For this review, use the dimensioned drawing (mm, ordinates from the lowest corner) and the shaded views. A direction names the side the tool comes from. Round coordinates to 2 decimals unless told otherwise and drop trailing zeros. Loops run counter-clockwise (first coordinate to the right, second up) from the corner with the lowest first, then second, coordinate; pieces in that order, holes last. Notation, with made-up numbers: M -3.75,42.25 L 49.25,42.25 A33 cw 49.25,79.25 Z; hole C 86.5,-36.5 d10. An arc over 180 degrees is marked long. One line per item, written item: value. Start each with the question number.
Item 1: For line 1 along Y through (x, z) = (5.5, 7.25); line 2 along X through (y, z) = (25.5, 5.5); line 3 along X through (y, z) = (42.5, 3.5), list the stretches that pass through material, from the lowest coordinate up.
Item 2: We need section A-A (z = 5.5). Write out the cut boundary in (x, y).
Item 3: We need section D-D (y = 42.5). Write out the cut boundary in (x, z).
Item 4: Clearance check with flat-ended pins moving along their axes: pin 1 (6 mm diameter, centred on y = 23, z = 8, fed in from +X); pin 2 (2 mm diameter, centred on y = 36, z = 2.5, fed in from +X); pin 3 (1.8 mm diameter, centred on x = 5.5, y = 42.5, fed in from -Z); pin 4 (3 mm diameter, centred on x = 1.5, y = 13, fed in from +Z). State where each tip first meets the part, or that it passes through.
Item 5: For the marked faces 1, 2 and 3, list the 3-axis set-ups (+Z, -Z, +X, -X, +Y, -Y) from which the entire face can be reached by the end or side of a thin tool; tool diameter is ignored.
Item 6: We need section B-B (x = 5.5). Write out the cut boundary in (y, z), then the cut area to 3 significant figures.
Item 7: We need section C-C (y = 11). Write out the cut boundary in (x, z).
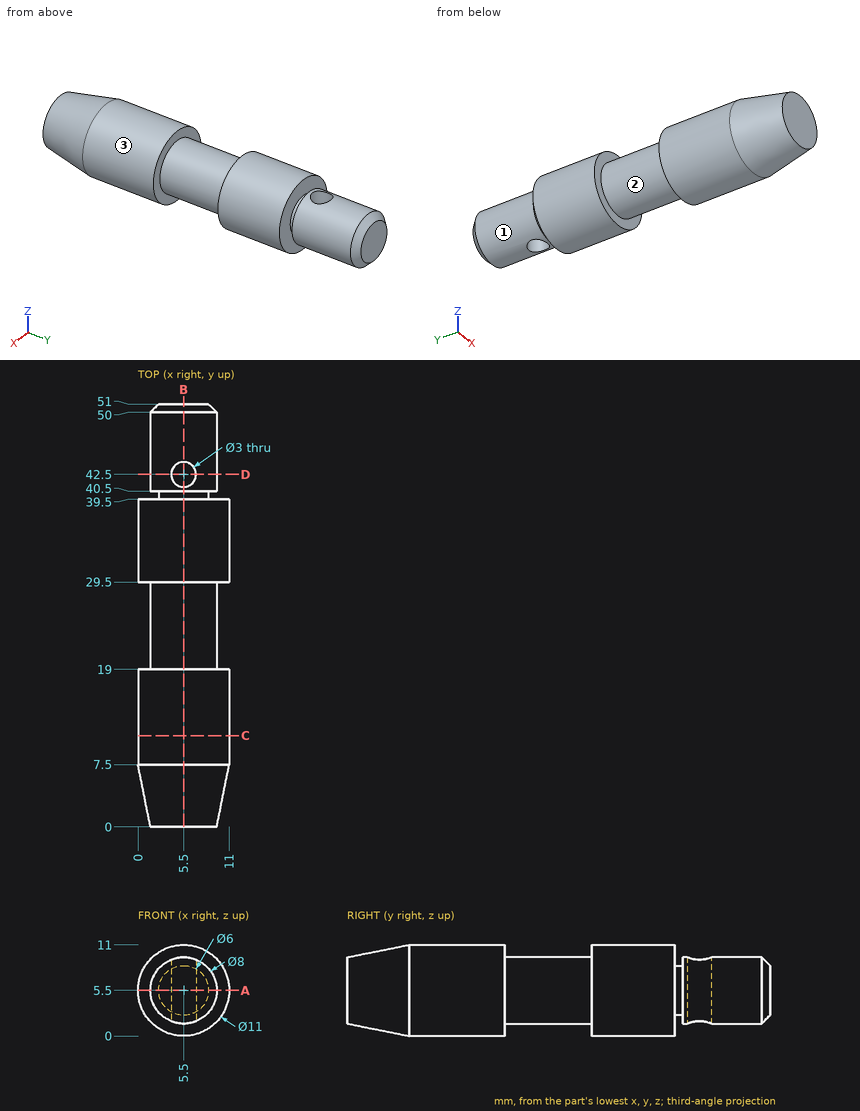
A:
1. line 1: 0 to 41, 44 to 51
1. line 2: 1.5 to 9.5
1. line 3: 2.04 to 4, 7 to 8.96
2. outline: M 0,7.5 L 1.5,0 L 9.5,0 L 11,7.5 L 11,19 L 9.5,19 L 9.5,29.5 L 11,29.5 L 11,39.5 L 8.5,39.5 L 8.5,40.5 L 9.5,40.5 L 9.5,50 L 8.5,51 L 2.5,51 L 1.5,50 L 1.5,40.5 L 2.5,40.5 L 2.5,39.5 L 0,39.5 L 0,29.5 L 1.5,29.5 L 1.5,19 L 0,19 Z; hole C 5.5,42.5 d3
3. outline: M 4,1.79 L 4,9.21 A4 ccw Z; M 7,1.79 A4 ccw 7,9.21 Z
4. pin 1: x = 9.5
4. pin 2: x = 10.62
4. pin 3: through
4. pin 4: z = 10.4
5. face 1: +Y
5. face 2: none
5. face 3: +Y, -Y
6. outline: M 0,1.5 L 7.5,0 L 19,0 L 19,1.5 L 29.5,1.5 L 29.5,0 L 39.5,0 L 39.5,2.5 L 40.5,2.5 L 40.5,1.5 L 41,1.5 L 41,9.5 L 40.5,9.5 L 40.5,8.5 L 39.5,8.5 L 39.5,11 L 29.5,11 L 29.5,9.5 L 19,9.5 L 19,11 L 7.5,11 L 0,9.5 Z; M 44,1.5 L 50,1.5 L 51,2.5 L 51,8.5 L 50,9.5 L 44,9.5 Z
6. area: 457 mm2
7. outline: C 5.5,5.5 d11
